Autodesk Inventor part; units mm, degrees
ref_plane "YZ Plane" through (0, 0, 0) normal (1, 0, 0) x (0, 1, 0)
ref_plane "XZ Plane" through (0, 0, 0) normal (0, 1, 0) x (-1, 0, 0)
ref_plane "XY Plane" through (0, 0, 0) normal (0, 0, 1) x (1, 0, 0)
sketch "Sketch1" plane through (0, 0, 0) normal (1, 0, 0) x (0, 1, 0)
  line L0 (0, 0) -> (16, 0)
  line L1 (16, 0) -> (16, 26)
  line L2 (16, 26) -> (0, 26)
  line L3 (0, 26) -> (0, 0)
  circle A0 centre (8, 18) radius 4
  dimension "d0" = 16
  dimension "d1" = 26
  dimension "d4" = 8
extrude "Extrusion1" add sketch "Sketch1" along normal blind 16
sketch "Sketch2" plane through (0, 16, 26) normal (0, 1, 0) x (1, 0, 0)
  circle A0 centre (8, 18) radius 4
  dimension "d8" = 8
extrude "Extrusion2" cut sketch "Sketch2" against normal blind 16
properties part number "BarClamp" material "Birch"
The model under review builds one solid part; all positions refer to its coordinate system, in mm. Round coordinates to 2 decimals unless told otherwise and drop trailing zeros. Loops run counter-clockwise (first coordinate to the right, second up) from the corner with the lowest first, then second, coordinate; pieces in that order, holes last. Notation, with made-up numbers: (16, 21.25) - (36, 21.25) arc R19 cw to (36, 27.25) - close; hole circle Ø1 at (83, 10.5). An arc over 180 degrees is marked (long way). Use CSV: the item, a comma, the result in double quotes.
(1) Take a section at D-D, the plane x = 2.75. Give the boundary of the cut face in (y, z), plus the area to 3 significant figures.
Working result:
outline,"(0, 0) - (16, 0) - (16, 26) - (0, 26) - close; hole circle Ø8 at (8, 18)"
area,"366 mm^2"
(2) Take a section at C-C, the plane z = 18. Give the boundary of the cut face in (x, y).
Working result:
outline,"(0, 0) - (16, 0) - (16, 4) - (0, 4) - close; (0, 12) - (16, 12) - (16, 16) - (0, 16) - close"
(3) Take a section at A-A, the plane x = 8. Give the boundary of the cut face in (y, z), plus the area to 3 significant figures.
Working result:
outline,"(0, 0) - (16, 0) - (16, 4) - (0, 4) - close; (0, 12) - (16, 12) - (16, 26) - (0, 26) - close; hole circle Ø8 at (8, 18)"
area,"238 mm^2"
(4) For line 1 (X direction, y = 4.25, z = 8); line 2 (Z direction, x = 8, y = 11); line 3 (Z direction, x = 4.5, y = 5.25), list the stretches that pass through material, from the lowest coordinate up.
Working result:
line 1,"x = 0 to 4, 12 to 16"
line 2,"z = 0 to 4, 12 to 15.35, 20.65 to 26"
line 3,"z = 0 to 6.06, 9.94 to 15.1, 20.9 to 26"
(5) Take a section at B-B, the plane y = 8. Give the boundary of the cut face in (x, z), plus the area to 3 significant figures.
Working result:
outline,"(0, 0) - (16, 0) - (16, 14) - (0, 14) - close; (0, 22) - (16, 22) - (16, 26) - (0, 26) - close; hole circle Ø8 at (8, 8)"
area,"238 mm^2"
(6) The part is to be moulded in two halves that separate along Y. For faces 1 (the cylindrical face through (7.89, 5.05, 15.3)), 2 (the flat face through (8, 16, 13)), 3 (the flat face through (8, 8, 26)), 4 (the flat face through (8, 0, 13)), say which applies: pulls with the +Y half, pulls with the -Y half, needs draft (parallel to the pull), parting line crosses it, or undercut.
Working result:
face 1,"undercut"
face 2,"pulls with the +Y half"
face 3,"needs draft"
face 4,"pulls with the -Y half"
